Autodesk Inventor part; units mm, degrees
ref_plane "YZ Plane" through (0, 0, 0) normal (1, 0, 0) x (0, 1, 0)
ref_plane "XZ Plane" through (0, 0, 0) normal (0, 1, 0) x (-1, 0, 0)
ref_plane "XY Plane" through (0, 0, 0) normal (0, 0, 1) x (1, 0, 0)
sketch "Sketch1" plane through (0, 0, 0) normal (0, 1, 0) x (-1, 0, 0)
  line L0 (76, 19) -> (-76, 19)
  line L1 (-76, 19) -> (-76, -19)
  line L2 (-76, -19) -> (76, -19)
  line L3 (76, -19) -> (76, 19)
  line L4 (76, 19) -> (-76, -19) construction
  line L5 (-76, 19) -> (76, -19) construction
  point P0 (0, 0)
  dimension "d0" = 152
  dimension "d1" = 38
extrude "Extrusion1" add sketch "Sketch1" along normal blind 2
sketch "Sketch2" plane through (0, 0, 0) normal (0, -1, 0) x (1, 0, 0)
  line L0 (76, 19) -> (76, -19)
  line L1 (-76, 19) -> (76, 19)
  line L2 (-76, -19) -> (-76, 19)
  line L3 (76, -19) -> (-76, -19)
  line L4 (-76, -19) -> (-76, 19)
  line L5 (-76, 19) -> (76, 19)
  line L6 (-76, -19) -> (76, -19)
  line L7 (76, -19) -> (76, 19)
  line L8 (76, 19) -> (-76, 19)
  line L9 (-76, 19) -> (-76, -19)
  line L10 (-76, -19) -> (-75.15, -19)
  line L11 (76, -19) -> (-76, -19)
  line L12 (76, 19) -> (76, 18.15)
  line L13 (76, 19) -> (76, -19)
  line L14 (-74.85, -18.35) -> (74.85, -18.35)
  line L15 (75.35, -17.85) -> (75.35, 17.85)
  line L16 (74.85, 18.35) -> (-74.85, 18.35)
  line L17 (-75.35, 17.85) -> (-75.35, -17.85)
  line L18 (75.35, -18.35) -> (74.4, -18.35)
  line L19 (-75.35, 18.35) -> (-74.4, 18.35)
  line L20 (73.35, -16.85) -> (-73.35, -16.85)
  line L21 (-73.85, -16.35) -> (-73.85, 16.35)
  line L22 (-73.35, 16.85) -> (73.35, 16.85)
  line L23 (73.85, 16.35) -> (73.85, -16.35)
  arc A0 (-74.85, 18.35) -> (-75.35, 17.85) centre (-74.85, 17.85) ccw
  arc A1 (-73.35, 16.85) -> (-73.85, 16.35) centre (-73.35, 16.35) ccw
  arc A2 (-75.35, -17.85) -> (-74.85, -18.35) centre (-74.85, -17.85) ccw
  arc A3 (-73.85, -16.35) -> (-73.35, -16.85) centre (-73.35, -16.35) ccw
  arc A4 (73.35, -16.85) -> (73.85, -16.35) centre (73.35, -16.35) ccw
  arc A5 (74.85, -18.35) -> (75.35, -17.85) centre (74.85, -17.85) ccw
  arc A6 (73.85, 16.35) -> (73.35, 16.85) centre (73.35, 16.35) ccw
  arc A7 (75.35, 17.85) -> (74.85, 18.35) centre (74.85, 17.85) ccw
  point P0 (0, 0)
  point P1 (-75.35, -18.35)
  point P2 (75.35, 18.35)
  point P3 (73.85, -16.85)
  point P4 (-73.85, 16.85)
  point P5 (-73.85, -16.85)
  point P6 (73.85, 16.85)
  dimension "d28" = 1.5
  dimension "d29" = 1.5
  dimension "d30" = 1.5
  dimension "d32" = 1.5
  dimension "d33" = 0.65
  dimension "d34" = 0.65
  dimension "d35" = 0.65
  dimension "d36" = 0.65
  dimension "d37" = 0.5
extrude "Extrusion2" cut sketch "Sketch2" against normal blind 0.75 contours A2 L17 A0 L16 A7 L15 A5 L14 | L20 A3 L21 A1 L22 A6 L23 A4
sketch "Sketch3" plane through (0, 0, 0) normal (0, -1, 0) x (1, 0, 0)
  line L0 (-74.85, 18.35) -> (74.85, 18.35)
  line L1 (-75.35, -17.85) -> (-75.35, 17.85)
  line L2 (74.85, -18.35) -> (-74.85, -18.35)
  line L3 (75.35, 17.85) -> (75.35, -17.85)
  line L4 (76, 19) -> (76, -19)
  line L5 (-76, 19) -> (76, 19)
  line L6 (-76, -19) -> (-76, 19)
  line L7 (76, -19) -> (-76, -19)
  line L8 (-75.35, -17.85) -> (-75.35, 17.85)
  line L9 (-74.85, 18.35) -> (74.85, 18.35)
  line L10 (75.35, 17.85) -> (75.35, -17.85)
  line L11 (74.85, -18.35) -> (-74.85, -18.35)
  line L12 (-73.85, 16.85) -> (-73.85, -16.85)
  line L13 (-73.85, -16.85) -> (73.85, -16.85)
  line L14 (73.85, -16.85) -> (73.85, 16.85)
  line L15 (73.85, 16.85) -> (-73.85, 16.85)
  line L16 (-73.85, 16.85) -> (-73.85, -16.85)
  line L17 (-73.85, 16.85) -> (-65.85, 16.85)
  line L18 (-65.85, 16.85) -> (-65.85, 8.85)
  line L19 (-65.85, 8.85) -> (-73.85, 8.85)
  line L20 (-73.85, 8.85) -> (-73.85, 16.85)
  line L21 (-73.85, -16.85) -> (-65.85, -16.85)
  line L22 (-65.85, -16.85) -> (-65.85, -8.85)
  line L23 (-65.85, -8.85) -> (-73.85, -8.85)
  line L24 (-73.85, -8.85) -> (-73.85, -16.85)
  line L25 (73.85, -16.85) -> (73.85, 16.85)
  line L26 (73.85, 16.85) -> (65.85, 16.85)
  line L27 (65.85, 16.85) -> (65.85, 8.85)
  line L28 (65.85, 8.85) -> (73.85, 8.85)
  line L29 (73.85, 8.85) -> (73.85, 16.85)
  line L30 (-73.85, -16.85) -> (73.85, -16.85)
  line L31 (73.85, -16.85) -> (65.85, -16.85)
  line L32 (65.85, -16.85) -> (65.85, -8.85)
  line L33 (65.85, -8.85) -> (73.85, -8.85)
  line L34 (73.85, -8.85) -> (73.85, -16.85)
  line L35 (-73.85, -16.85) -> (-65.85, -8.85)
  line L36 (-65.85, -16.85) -> (-73.85, -8.85)
  line L37 (-73.85, 8.85) -> (-65.85, 16.85)
  line L38 (73.85, 16.85) -> (-73.85, 16.85)
  line L39 (-65.85, 8.85) -> (-73.85, 16.85)
  circle A0 centre (-69.85, -12.85) radius 1.65
  circle A1 centre (-69.85, 12.85) radius 1.65
  line L40 (65.85, -16.85) -> (73.85, -8.85)
  line L41 (65.85, 8.85) -> (73.85, 16.85)
  line L42 (73.85, 8.85) -> (65.85, 16.85)
  line L43 (73.85, -16.85) -> (65.85, -8.85)
  circle A2 centre (69.85, -12.85) radius 1.65
  circle A3 centre (69.85, 12.85) radius 1.65
  arc A4 (-75.35, -17.85) -> (-74.85, -18.35) centre (-74.85, -17.85) ccw
  arc A5 (-74.85, 18.35) -> (-75.35, 17.85) centre (-74.85, 17.85) ccw
  arc A6 (75.35, 17.85) -> (74.85, 18.35) centre (74.85, 17.85) ccw
  arc A7 (74.85, -18.35) -> (75.35, -17.85) centre (74.85, -17.85) ccw
  arc A8 (-75.35, -17.85) -> (-74.85, -18.35) centre (-74.85, -17.85) ccw
  arc A9 (74.85, -18.35) -> (75.35, -17.85) centre (74.85, -17.85) ccw
  arc A10 (75.35, 17.85) -> (74.85, 18.35) centre (74.85, 17.85) ccw
  arc A11 (-74.85, 18.35) -> (-75.35, 17.85) centre (-74.85, 17.85) ccw
  point P0 (0, 0)
  dimension "d14" = 8
  dimension "d15" = 8
  dimension "d16" = 8
  dimension "d17" = 8
  dimension "d18" = 8
  dimension "d19" = 8
  dimension "d20" = 8
  dimension "d21" = 8
  dimension "d22" = 3.3
  dimension "d23" = 3.3
  dimension "d24" = 3.3
  dimension "d25" = 3.3
extrude "Extrusion3" cut sketch "Sketch3" against normal blind 3 contours A1 L37 L39 | L39 L37 A1 | L37 L39 A1 | A1 L39 L37 | A0 L35 L36 | L36 L35 A0 | A3 L41 L42 | L42 L41 A3 | L35 L36 A0 | A0 L36 L35 | A3 L42 L41 | L41 L42 A3 | A2 L43 L40 | L40 L43 A2 | A2 L43 L40 | L40 L43 A2
sketch "Sketch4" plane through (0, 0, 0) normal (0, -1, 0) x (1, 0, 0)
  point P0 (0, 0)
properties part number "tapa" material "Steel, Mild, Welded"
Geometry check sheet. Reference: the model listing, model coordinates, mm. A direction names the side the tool comes from. Give positions to 0.01 mm unless a question says otherwise; leave off trailing zeros. Loops run counter-clockwise (first coordinate to the right, second up) from the corner with the lowest first, then second, coordinate; pieces in that order, holes last. Notation, with made-up numbers: M 64.5,89 L 89.5,89 A22 cw 89.5,127 Z; hole C 70.25,62.25 d7. An arc over 180 degrees is marked long. Write each question's results on one line, items separated by ' | '.
1) Release check for a two-part mould opening along X. For faces 1 (the face through (-68.326, 1.366, -13.482)), 2 (the face through (1, 2, 0)) record: +X half, -X half, draft (parallel to the pull), parting line (faces both ways), or undercut.
Answers follow:
face 1: undercut | face 2: draft
2) Section check D-D, the plane z = -1. Record the boundary of the cut face in (x, y), plus the area to 3 significant figures.
Answers follow:
outline: M -76,0 L -75.35,0 L -75.35,0.75 L 75.35,0.75 L 75.35,0 L 76,0 L 76,2 L -76,2 Z | area: 191 mm2
3) Section check A-A, the plane x = -69.85. Record the boundary of the cut face in (y, z), plus the area to 3 significant figures.
Answers follow:
outline: M 0,-19 L 2,-19 L 2,-14.5 L 0.75,-14.5 L 0.75,-18.35 L 0,-18.35 Z; M 0,18.35 L 0.75,18.35 L 0.75,14.5 L 2,14.5 L 2,19 L 0,19 Z; M 0.75,-11.2 L 2,-11.2 L 2,11.2 L 0.75,11.2 Z | area: 40.2 mm2
4) Tool access check on faces 3 (the face through (-68.326, 1.366, 12.218)), 4 (the face through (-1, 0.75, 0)). Record the directions out of +Z, -Z, +X, -X, +Y, -Y that give a thin tool (end or side, any length) a straight path to the whole face; none if there is none.
Answers follow:
face 3: +Y, -Y | face 4: -Y
5) Section check C-C, the plane y = 0.3. Record the boundary of the cut face in (x, z), plus the area to 3 significant figures.
Answers follow:
outline: M -76,-19 L 76,-19 L 76,19 L -76,19 Z; hole M -75.35,-17.85 A0.5 ccw -74.85,-18.35 L 74.85,-18.35 A0.5 ccw 75.35,-17.85 L 75.35,17.85 A0.5 ccw 74.85,18.35 L -74.85,18.35 A0.5 ccw -75.35,17.85 Z | area: 246 mm2
6) Gauge pin test, flat ends, axial feed: pin 1 (8 mm diameter, centred on x = 5.5, z = 2, fed in from -Y); pin 2 (3 mm diameter, centred on x = 69.85, z = 12.85, fed in from -Y). Record the tip position at first contact, or that the pin passes through.
Answers follow:
pin 1: y = 0.75 | pin 2: through
7) Thickness scan on line 1 (Z direction, x = 69.85, y = 1.55); line 2 (Z direction, x = 66, y = 0.65); line 3 (X direction, y = 0.7, z = -1). Record the ranges inside material, lowest first.
Answers follow:
line 1: -19 to -14.5, -11.2 to 11.2, 14.5 to 19 | line 2: -19 to -18.35, 18.35 to 19 | line 3: -76 to -75.35, 75.35 to 76
8) Section check B-B, the plane z = 12.85. Record the boundary of the cut face in (x, y).
Answers follow:
outline: M -76,0 L -75.35,0 L -75.35,0.75 L -71.5,0.75 L -71.5,2 L -76,2 Z; M -68.2,0.75 L 68.2,0.75 L 68.2,2 L -68.2,2 Z; M 71.5,0.75 L 75.35,0.75 L 75.35,0 L 76,0 L 76,2 L 71.5,2 Z
